Model file for the job. Use its own axes, mm. Face numbers are marked on the shaded views. A direction names the side the tool comes from. Round coordinates to 2 decimals unless told otherwise and drop trailing zeros. Loops run counter-clockwise (first coordinate to the right, second up) from the corner with the lowest first, then second, coordinate; pieces in that order, holes last. Notation, with made-up numbers: (-16, 18) -> (0, 18) arc R17 ccw to (0, 28) -> close; hole circle Ø5 at (-37.75, -0.5). An arc over 180 degrees is marked (long way). Use a Markdown table: item, result.
from build123d import *

# Parameters (mm, degrees)
BOSS_EXTRUDE2_DEPTH = 10


with BuildPart() as part:
    # Sketch1 → Boss-Extrude2 (new body)
    with BuildSketch(Plane.XY):
        Polygon((9.945212763, 7.004832947), (8.692356553, 10.417594294), (5.110390425, 11.038969663), (2.319004447, 13.368079582), (-1.0937569, 12.115223372), (-4.675723029, 12.736598741), (-7.004832947, 9.945212763), (-10.417594294, 8.692356553), (-11.038969663, 5.110390425), (-13.368079582, 2.319004447), (-12.115223372, -1.0937569), (-12.736598741, -4.675723029), (-9.945212763, -7.004832947), (-8.692356553, -10.417594294), (-5.110390425, -11.038969663), (-2.319004447, -13.368079582), (1.0937569, -12.115223372), (4.675723029, -12.736598741), (7.004832947, -9.945212763), (10.417594294, -8.692356553), (11.038969663, -5.110390425), (13.368079582, -2.319004447), (12.115223372, 1.0937569), (12.736598741, 4.675723029), align=None)
        with BuildLine():
            Line((-3.08920951, -4.05792861), (-2.537148142, 4.424124694))
            ThreePointArc((-2.537148142, 4.424124694), (5.089231982, -0.331236821), (-3.08920951, -4.05792861))
        make_face(mode=Mode.SUBTRACT)
    extrude(amount=BOSS_EXTRUDE2_DEPTH)


solid = part.part
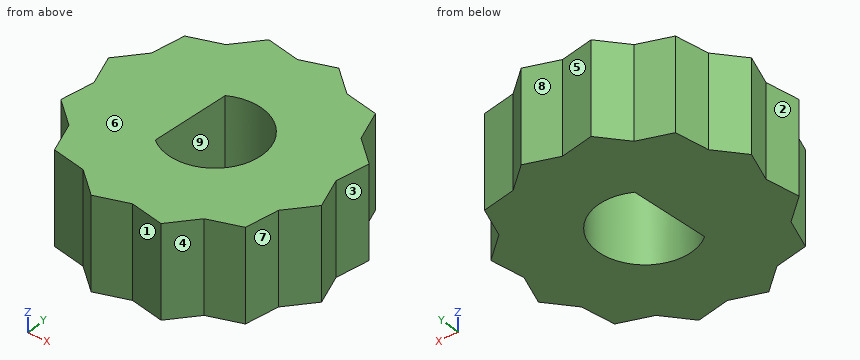
Q1. Tool access for the marked faces 1, 2, 3, 4 and 5: list every direction of +Z, -Z, +X, -X, +Y, -Y with a clear straight run to the whole face (end or side of a thin tool).
Results list:
| item | result |
|---|---|
| face 1 | +Z, -Z, -Y |
| face 2 | +Z, -Z, -X |
| face 3 | +Z, -Z, +X |
| face 4 | +Z, -Z, +X, -Y |
| face 5 | +Z, -Z, +Y |
Q2. Band-saw the part on A-A, the plane z = 2.25. Give the cut face in (x, y), plus the area to 3 significant figures.
Results list:
| item | result |
|---|---|
| outline | (-13.37, 2.32) -> (-12.12, -1.09) -> (-12.74, -4.68) -> (-9.95, -7) -> (-8.69, -10.42) -> (-5.11, -11.04) -> (-2.32, -13.37) -> (1.09, -12.12) -> (4.68, -12.74) -> (7, -9.95) -> (10.42, -8.69) -> (11.04, -5.11) -> (13.37, -2.32) -> (12.12, 1.09) -> (12.74, 4.68) -> (9.95, 7) -> (8.69, 10.42) -> (5.11, 11.04) -> (2.32, 13.37) -> (-1.09, 12.12) -> (-4.68, 12.74) -> (-7, 9.95) -> (-10.42, 8.69) -> (-11.04, 5.11) -> close; hole (-3.09, -4.06) arc R5.1 ccw (long way) to (-2.54, 4.42) -> close |
| area | 445 mm² |
Q3. Band-saw the part on B-B, the plane y = 0. Give the cut face in (x, z).
Results list:
| item | result |
|---|---|
| outline | (-12.52, 0) -> (-2.83, 0) -> (-2.83, 10) -> (-12.52, 10) -> close; (5.1, 0) -> (12.52, 0) -> (12.52, 10) -> (5.1, 10) -> close |
Q4. Flat gauge pins, fed straight in: pin 1 (4 mm diameter, centred on x = 1.5, z = 2.5, fed in from -Y); pin 2 (2 mm diameter, centred on x = -7, z = 8, fed in from +Y); pin 3 (5 mm diameter, centred on y = 8, z = 6, fed in from -X). Where does each tip first touch, or does it go through?
Results list:
| item | result |
|---|---|
| pin 1 | stops at y = -12.7 |
| pin 2 | stops at y = 11.15 |
| pin 3 | stops at x = -10.97 |
Q5. Drill centre lines: L1, parallel to Y at x = 0, z = 4.25; L2, parallel to X at y = 0, z = 4.5; L3, parallel to X at y = -2, z = 1. Where is each one in solid material? Low to high. Write a range as from..to.
Results list:
| item | result |
|---|---|
| L1 | y = -12.52..-5.1, 5.1..12.52 |
| L2 | x = -12.52..-2.83, 5.1..12.52 |
| L3 | x = -12.27..-2.96, 4.69..13.25 |
Q6. Band-saw the part on C-C, the plane x = 0. Give the cut face in (y, z), plus the area to 3 significant figures.
Results list:
| item | result |
|---|---|
| outline | (-12.52, 0) -> (-5.1, 0) -> (-5.1, 10) -> (-12.52, 10) -> close; (5.1, 0) -> (12.52, 0) -> (12.52, 10) -> (5.1, 10) -> close |
| area | 148 mm² |
Q7. Pull direction Y, two halves, no side cores. Call the marked faces 6, 7, 8 and 9: released by +Y, released by -Y, zero draft, split by the parting line, or undercut.
Results list:
| item | result |
|---|---|
| face 6 | zero draft |
| face 7 | released by -Y |
| face 8 | released by +Y |
| face 9 | undercut |
Q8. Band-saw the part on D-D, the plane y = 8. Give the cut face in (x, z).
Results list:
| item | result |
|---|---|
| outline | (-10.54, 0) -> (9.58, 0) -> (9.58, 10) -> (-10.54, 10) -> close |
